Source: three-view drawing plus pictorial views. Frame: mm from the lowest corner of the part. A direction names the side the tool comes from. Round coordinates to 2 decimals unless told otherwise and drop trailing zeros. Order: outer loops, then holes, each group sorted by start corner. A loop starts at its lowest first (then second) coordinate and runs counter-clockwise, first axis right, second up. Notation, with made-up numbers: (32, 21) -> (82, 21) arc R22 ccw to (82, 55) -> close; hole circle Ø9 at (43.25, 88). An arc over 180 degrees is marked (long way). Use a Markdown table: item, result.
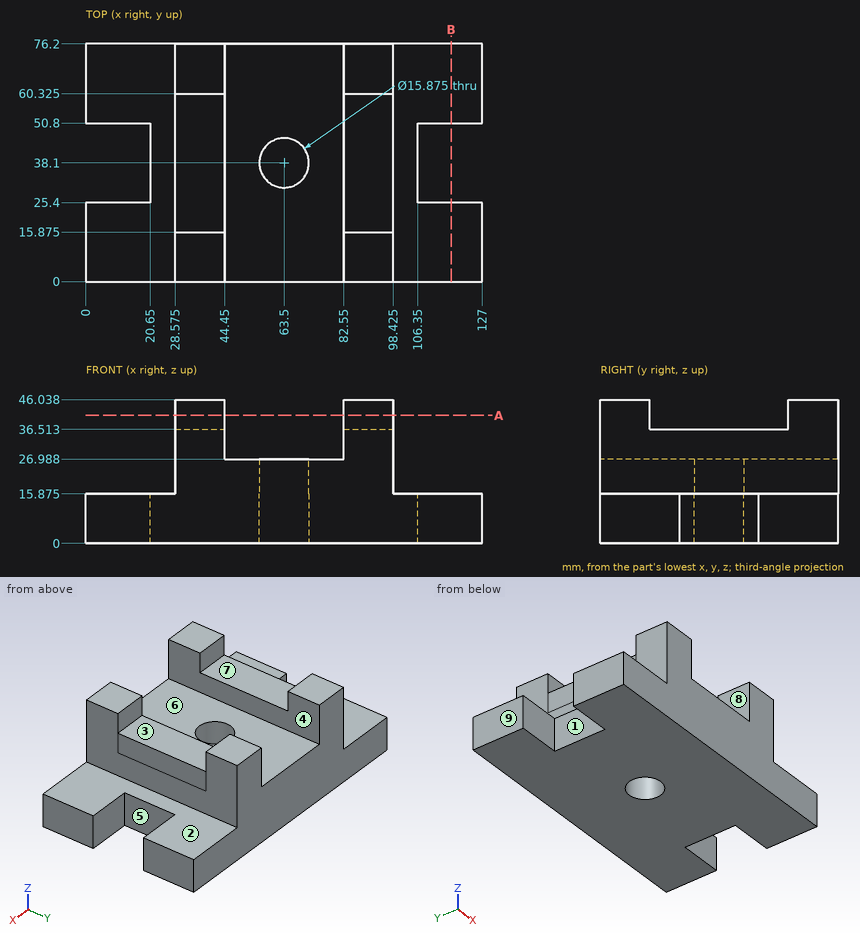
1) Line query: L1, parallel to Y at x = 63.5, z = 21.25; L2, parallel to X at y = 38, z = 9; L3, parallel to Y at x = 96.5, z = 43 (1 decimal). Output: solid intervals per line, ascending. Write a range as [from, to].
Results found:
| item | result |
|---|---|
| L1 | y = [0, 30.16], [46.04, 76.2] |
| L2 | x = [20.65, 55.56], [71.44, 106.35] |
| L3 | y = [0, 15.9], [60.3, 76.2] |
2) Cut plane A-A on z = 41. Count the separate pieces of the cut face and the enclosed holes in it, and give its area (3 significant figures).
Results found:
| item | result |
|---|---|
| separate pieces | 4 |
| enclosed holes | 0 |
| area | 1,010 mm² |
3) Cut plane B-B on x = 117. Return loops of the section in (y, z) (1 decimal).
Results found:
| item | result |
|---|---|
| outline | (0, 0) -> (25.4, 0) -> (25.4, 15.9) -> (0, 15.9) -> close; (50.8, 0) -> (76.2, 0) -> (76.2, 15.9) -> (50.8, 15.9) -> close |
4) Pull-direction query (X, two-part tool) for the marked faces 6, 7, 8 and 9; classes: +X half, -X half, draft (parallel to the pull), parting line (faces both ways), or undercut.
Results found:
| item | result |
|---|---|
| face 6 | undercut |
| face 7 | draft |
| face 8 | undercut |
| face 9 | -X half |
5) Pin query (flat end, axial travel): pin 1 Ø1.5 at (x, y) = (64.5, 60.5) entering from -Z; pin 2 Ø2 at (y, z) = (35, 18) entering from -X (1 decimal); pin 3 Ø3 at (y, z) = (68, 26.5) entering from +X (1 decimal); pin 4 Ø8 at (x, y) = (40, 36.5) entering from +Z. Return the tip coordinate at first contact, or that it passes through.
Results found:
| item | result |
|---|---|
| pin 1 | stops at z = 0 |
| pin 2 | stops at x = 28.6 |
| pin 3 | stops at x = 98.4 |
| pin 4 | stops at z = 36.51 |
6) Set-up query: the marked faces 1, 2, 3, 4 and 5. Return all of +Z, -Z, +X, -X, +Y, -Y with unobstructed straight access to the full face (end or side cutting, diameter ignored); none if empty.
Results found:
| item | result |
|---|---|
| face 1 | +Z, -Z, -X |
| face 2 | +Z, +X, +Y, -Y |
| face 3 | +Z, +X, -X |
| face 4 | +Z, +Y, -Y |
| face 5 | +Z, -Z, +X |
